Could you check a few things on this model? Use its own coordinates, in mm. Round coordinates to 2 decimals unless told otherwise and drop trailing zeros. Loops run counter-clockwise (first coordinate to the right, second up) from the corner with the lowest first, then second, coordinate; pieces in that order, holes last. Notation, with made-up numbers: (40, 31) -> (58, 31) arc R11 cw to (58, 50) -> close; hole circle Ø5 at (-25, 58.25). An arc over 180 degrees is marked (long way). One line per item, written item: value.
```python
from build123d import *

# Parameters (mm, degrees)
SKETCH1_W           = 100
SKETCH1_H           = 50
BOSS_EXTRUDE1_DEPTH = 20
SKETCH2_R           = 15
CUT_EXTRUDE1_DEPTH  = 20
FILLET1_R           = 10
CHAMFER1_SIZE       = 1


with BuildPart() as part:
    # Sketch1 → Boss-Extrude1 (new body)
    with BuildSketch(Plane(origin=(0, 0, 0), x_dir=(1, 0, 0), z_dir=(0, 1, 0))):
        Rectangle(SKETCH1_W, SKETCH1_H)
    extrude(amount=BOSS_EXTRUDE1_DEPTH)

    # Sketch2 → Cut-Extrude1 (cut)
    with BuildSketch(Plane(origin=(0, 20, 0), x_dir=(1, 0, 0), z_dir=(0, 1, 0))):
        with Locations(Location((0, 0, 0), (0, 0, 270))):
            Circle(SKETCH2_R)
    extrude(amount=-CUT_EXTRUDE1_DEPTH, mode=Mode.SUBTRACT)

    # Fillet1
    fillet1_edges = [part.edges().sort_by_distance(p)[0] for p in [
        (50, 10, 25),
        (-50, 10, 25),
        (50, 10, -25),
    ]]
    fillet(fillet1_edges, radius=FILLET1_R)

    # Chamfer1
    chamfer1_edges = [part.edges().sort_by_distance(p)[0] for p in [
        (-50, 20, -5),
        (-5, 20, -25),
        (50, 20, 0),
        (0, 20, 25),
        (-47.071067812, 20, 22.071067812),
        (47.071067812, 20, 22.071067812),
        (47.071067812, 20, -22.071067812),
    ]]
    chamfer(chamfer1_edges, length=CHAMFER1_SIZE)


solid = part.part
```
Item 1: I need wall thicknesses on line 1 (X direction, y = 12, z = 0); line 2 (Z direction, x = 7, y = 17.75); line 3 (X direction, y = 9.5, z = 10). Which ranges of each line are inside material? Lowest first, please. Write a range as from..to.
Output:
line 1: x = -50..-15, 15..50
line 2: z = -25..-13.27, 13.27..25
line 3: x = -50..-11.18, 11.18..50
Item 2: If we section it at A-A on z = 0: List the corners of the cut face in (x, y) for me.
Output:
outline: (-50, 0) -> (-15, 0) -> (-15, 20) -> (-49, 20) -> (-50, 19) -> close; (15, 0) -> (50, 0) -> (50, 19) -> (49, 20) -> (15, 20) -> close
Item 3: If we section it at C-C on y = 2.25: List the corners of the cut face in (x, z) for me, plus the area to 3 significant figures.
Output:
outline: (-50, -25) -> (40, -25) arc R10 ccw to (50, -15) -> (50, 15) arc R10 ccw to (40, 25) -> (-40, 25) arc R10 ccw to (-50, 15) -> close; hole circle Ø30 at (0, 0)
area: 4,230 mm²
Item 4: If we mould it in two halves opening along X, with no side actions, what happens to faces 1 (the face through (46.99, 9.63, 22.15)), 2 (the face through (0.66, 10.14, -14.985)), 3 (the face through (-50, 9, -5)), 4 (the face through (-12, 20, -11))? For each: released by +X, released by -X, zero draft, split by the parting line, or undercut.
Output:
face 1: released by +X
face 2: undercut
face 3: released by -X
face 4: zero draft
Item 5: If we section it at B-B on x = 0: List the corners of the cut face in (y, z) for me, plus the area to 3 significant figures.
Output:
outline: (0, -25) -> (19, -25) -> (20, -24) -> (20, -15) -> (0, -15) -> close; (0, 15) -> (20, 15) -> (20, 24) -> (19, 25) -> (0, 25) -> close
area: 399 mm²
